Input: part model. Units: mm. Frame: model coordinates. Face numbers are marked on the shaded views. A direction names the side the tool comes from. Coordinates: 2 decimals unless noted, no trailing zeros. Order: outer loops, then holes, each group sorted by start corner. A loop starts at its lowest first (then second) coordinate and runs counter-clockwise, first axis right, second up.
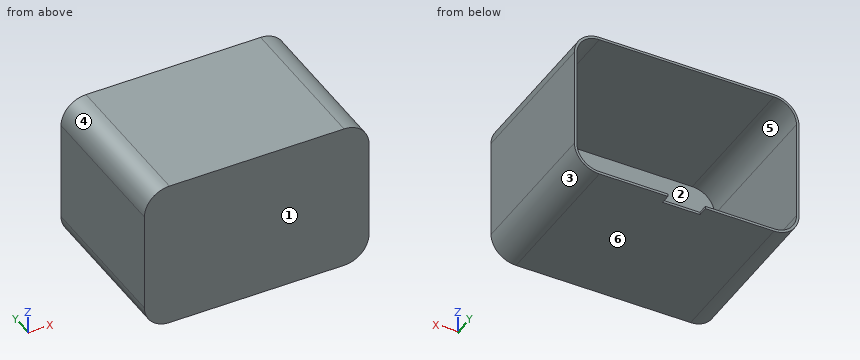
from build123d import *

# Parameters (mm, degrees)
EXTRUDE_1_DEPTH     = 1.2
EXTRUDE_2_DEPTH     = 60
SKETCH_5_W          = 15
SKETCH_5_H          = 8
CUT_EXTRUDE_1_DEPTH = 1.5


with BuildPart() as part:
    # 草图1 → 凸台-拉伸1 (new body)
    with BuildSketch(Plane(origin=(0, 0, 0), x_dir=(1, 0, 0), z_dir=(0, 1, 0))):
        with BuildLine():
            Line((-35, 30), (35, 30))
            ThreePointArc((35, 30), (42.071067812, 27.071067812), (45, 20))
            Line((45, 20), (45, -20))
            ThreePointArc((45, -20), (42.071067812, -27.071067812), (35, -30))
            Line((35, -30), (-35, -30))
            ThreePointArc((-35, -30), (-42.071067812, -27.071067812), (-45, -20))
            Line((-45, -20), (-45, 20))
            ThreePointArc((-45, 20), (-42.071067812, 27.071067812), (-35, 30))
        make_face()
    extrude(amount=EXTRUDE_1_DEPTH)

    # 草图2 → 凸台-拉伸2 (add)
    with BuildSketch(Plane(origin=(0, 1.2, 0), x_dir=(1, 0, 0), z_dir=(0, 1, 0))):
        with BuildLine():
            Line((45, -20), (45, 20))
            ThreePointArc((45, 20), (42.071067812, 27.071067812), (35, 30))
            Line((35, 30), (-35, 30))
            ThreePointArc((-35, 30), (-42.071067812, 27.071067812), (-45, 20))
            Line((-45, 20), (-45, -20))
            ThreePointArc((-45, -20), (-42.071067812, -27.071067812), (-35, -30))
            Line((-35, -30), (35, -30))
            ThreePointArc((35, -30), (42.071067812, -27.071067812), (45, -20))
        make_face()
        with BuildLine():
            Line((44, -20), (44, 20))
            ThreePointArc((44, 20), (41.363961031, 26.363961031), (35, 29))
            Line((35, 29), (-35, 29))
            ThreePointArc((-35, 29), (-41.363961031, 26.363961031), (-44, 20))
            Line((-44, 20), (-44, -20))
            ThreePointArc((-44, -20), (-41.363961031, -26.363961031), (-35, -29))
            Line((-35, -29), (35, -29))
            ThreePointArc((35, -29), (41.363961031, -26.363961031), (44, -20))
        make_face(mode=Mode.SUBTRACT)
    extrude(amount=EXTRUDE_2_DEPTH)

    # 草图5 → 切除-拉伸1 (cut)
    with BuildSketch(Plane(origin=(0, 0, -30), x_dir=(-1, 0, 0), z_dir=(0, 0, -1))):
        with Locations((0, 61.2)):
            Rectangle(SKETCH_5_W, SKETCH_5_H)
    extrude(amount=-CUT_EXTRUDE_1_DEPTH, mode=Mode.SUBTRACT)


solid = part.part
Item 1: Pin query (flat end, axial travel): pin 1 Ø1.1 at (x, z) = (-3, -29.5) entering from +Y; pin 2 Ø12 at (y, z) = (44.5, -23.5) entering from +X; pin 3 Ø17.5 at (x, z) = (-4, 10.5) entering from +Y; pin 4 Ø1.1 at (y, z) = (60, -29.5) entering from -X. Return the tip coordinate at first contact, or that it passes through.
Response values:
pin 1: stops at y = 57.2
pin 2: stops at x = 45
pin 3: stops at y = 1.2
pin 4: stops at x = -39.46
Item 2: Cut plane B-B on x = -1.5. Return loops of the section in (y, z).
Response values:
outline: (0, -30) - (57.2, -30) - (57.2, -29) - (1.2, -29) - (1.2, 29) - (61.2, 29) - (61.2, 30) - (0, 30) - close
Item 3: Cut plane C-C on z = -7. Return loops of the section in (x, y), then the cut area to 3 significant figures.
Response values:
outline: (-45, 0) - (45, 0) - (45, 61.2) - (44, 61.2) - (44, 1.2) - (-44, 1.2) - (-44, 61.2) - (-45, 61.2) - close
area: 228 mm2
Item 4: Ray query, probe 1 along X at (y, z) = (33, -2); probe 2 along Z at (x, y) = (-21.5, 58.5); probe 3 along Y at (x, z) = (-23, -2). Return the intervals inside material, ascending.
Response values:
probe 1: x = -45 to -44, 44 to 45
probe 2: z = -30 to -29, 29 to 30
probe 3: y = 0 to 1.2
Item 5: Access query for the marked faces 5 and 6. Directions: +Z, -Z, +X, -X, +Y, -Y. A direction counts if a zero-diameter tool reaches every point of the face in a straight line with its end or side. Return the directions, or none.
Response values:
face 5: +Y
face 6: -Z, +X, -X, +Y, -Y
Item 6: Cut plane A-A on y = 14.5. Return loops of the section in (x, z), then the cut area to 3 significant figures.
Response values:
outline: (-45, -20) arc R10 ccw to (-35, -30) - (35, -30) arc R10 ccw to (45, -20) - (45, 20) arc R10 ccw to (35, 30) - (-35, 30) arc R10 ccw to (-45, 20) - close; hole (-44, -20) arc R9 ccw to (-35, -29) - (35, -29) arc R9 ccw to (44, -20) - (44, 20) arc R9 ccw to (35, 29) - (-35, 29) arc R9 ccw to (-44, 20) - close
area: 280 mm2
Item 7: Draft query along Z for the marked faces 1, 2, 3 and 4. Return one class per face: pulls with the +Z half, pulls with the -Z half, needs draft (parallel to the pull), parting line crosses it, or undercut.
Response values:
face 1: needs draft
face 2: undercut
face 3: pulls with the -Z half
face 4: pulls with the +Z half
